Design review of the part built by this model. Coordinates are the model's own, in mm. A direction names the side the tool comes from. Coordinates: 2 decimals unless noted, no trailing zeros. Write each loop counter-clockwise with the first axis right and the second up, starting at its lowest first coordinate (ties: lowest second). Pieces come first, ordered by that corner, then holes.
Q1. Machinability: for faces 1 (the face through (150, 61.784, 2)), 2 (the face through (-48, -80, 2)), 3 (the face through (12.291, 83, 2)), 4 (the face through (-40, 1, 0)), 5 (the face through (150, -61.784, 2)), which of the approach directions +Z, -Z, +X, -X, +Y, -Y give a long, thin tool a straight path to every point of the face, cutting with its end or side? Answer none if there is none.
Q2. Add section B-B, the plane x = 56. Give the boundary of the cut face in (y, z), plus the area to 3 significant figures.
Q3. Clearance check with flat-ended pins moving along their axes: pin 1 Ø2.5 at (x, z) = (112, 2.5) entering from -Y; pin 2 Ø1.4 at (x, z) = (-51, 3) entering from +Y; pin 3 Ø1.4 at (x, z) = (-18.5, 1.5) entering from +Y; pin 4 Ø2.5 at (y, z) = (-82.5, 3) entering from -X. State where each tip first meets the part, or that it passes through.
Q4. To check wall thickness, follow probe 1 along X at (y, z) = (-83.5, 4); probe 2 along Y at (x, z) = (21, 1.5); probe 3 along X at (y, z) = (-9, 3.7). State the ranges of each line that lie inside material, in increasing order.
Q5. Add section A-A, the plane y = 6. Give the boundary of the cut face in (x, z), plus the area to 3 significant figures.
Q6. The part is to be moulded in two halves that separate along X. For faces 6 (the face through (50, -80.6, 2)), 7 (the face through (-12.084, 100, 2)), 8 (the face through (-30, 97.7, 2)), say which applies: +X half, -X half, draft (parallel to the pull), parting line (faces both ways), or undercut.
from build123d import *

# Parameters (mm, degrees)
BOSS_EXTRUDE1_DEPTH = 4.6
CUT_EXTRUDE1_DEPTH  = 5.6


with BuildPart() as part:
    # Sketch1 → Boss-Extrude1 (new body)
    with BuildSketch(Plane.XY):
        Polygon((147.4, 61.783577493), (152, 61.783577493), (152, -61.783577493), (147.4, -61.783577493), (147.4, -97.7), (111.483577493, -97.7), (111.483577493, -102.3), (-12.083577493, -102.3), (-12.083577493, -97.7), (-48, -97.7), (-48, -61.783577493), (-52.6, -61.783577493), (-52.6, 61.783577493), (-48, 61.783577493), (-48, 97.7), (-12.083577493, 97.7), (-12.083577493, 102.3), (111.483577493, 102.3), (111.483577493, 97.7), (147.4, 97.7), align=None)
    extrude(amount=BOSS_EXTRUDE1_DEPTH)

    # Sketch2 → Cut-Extrude1 (cut, through all)
    with BuildSketch(Plane(origin=(0, 0, 0), x_dir=(-1, 0, 0), z_dir=(0, 0, -1))):
        Polygon((-134.9, -85.2), (-87.108698535, -85.2), (-87.108698535, -80.6), (-12.291301465, -80.6), (-12.291301465, -85.2), (35.5, -85.2), (35.5, -37.408698535), (30.9, -37.408698535), (30.9, 37.408698535), (35.5, 37.408698535), (35.5, 85.2), (-12.291301465, 85.2), (-12.291301465, 80.6), (-87.108698535, 80.6), (-87.108698535, 85.2), (-134.9, 85.2), (-134.9, 37.408698535), (-130.3, 37.408698535), (-130.3, -37.408698535), (-134.9, -37.408698535), align=None)
    extrude(amount=-CUT_EXTRUDE1_DEPTH, mode=Mode.SUBTRACT)


solid = part.part
Here are the results:
1. face 1: +Z, -Z, +X, +Y
1. face 2: +Z, -Z, -X, -Y
1. face 3: +Z, -Z
1. face 4: -Z, +X, -X, +Y, -Y
1. face 5: +Z, -Z, +X, -Y
2. outline: (-102.3, 0) - (-80.6, 0) - (-80.6, 4.6) - (-102.3, 4.6) - close; (80.6, 0) - (102.3, 0) - (102.3, 4.6) - (80.6, 4.6) - close
2. area: 200 mm2
3. pin 1: stops at y = -102.3
3. pin 2: stops at y = 61.78
3. pin 3: stops at y = 97.7
3. pin 4: stops at x = -48
4. probe 1: x = -48 to -35.5, 12.29 to 87.11, 134.9 to 147.4
4. probe 2: y = -102.3 to -80.6, 80.6 to 102.3
4. probe 3: x = -52.6 to -30.9, 130.3 to 152
5. outline: (-52.6, 0) - (-30.9, 0) - (-30.9, 4.6) - (-52.6, 4.6) - close; (130.3, 0) - (152, 0) - (152, 4.6) - (130.3, 4.6) - close
5. area: 200 mm2
6. face 6: undercut
6. face 7: -X half
6. face 8: draft
